Read the model definition and answer for the solid it produces. Units are mm, in the model's axes. A direction names the side the tool comes from. Coordinates: 2 decimals unless noted, no trailing zeros. Write each loop counter-clockwise with the first axis right and the second up, starting at its lowest first coordinate (ties: lowest second). Pieces come first, ordered by that corner, then holes. Notation, with made-up numbers: (-15.75, -29) -> (9.25, -29) arc R34 ccw to (9.25, 8) -> close; hole circle Ø10 at (-14, 41). An arc over 180 degrees is marked (long way). Use CSV: the item, a comma, the result in double quotes.
from build123d import *

# Parameters (mm, degrees)
BOSS_EXTRUDE2_DEPTH   = 22
BOSS_EXTRUDE3_DEPTH   = 64
SKETCH3_R             = 3
CUT_EXTRUDE1_DEPTH    = 65
SKETCH4_R             = 6
CUT_EXTRUDE2_DEPTH    = 52
M4_TAPPED_HOLE1_D     = 3.3
M4_TAPPED_HOLE1_DEPTH = 14
M4_TAPPED_HOLE1_TIP   = 0.991420021
SKETCH8_R             = 2.5
SKETCH8_R_2           = 1.5
CUT_EXTRUDE3_DEPTH    = 5
SKETCH9_R             = 1
CUT_EXTRUDE4_DEPTH    = 15
CHAMFER1_SIZE         = 1


with BuildPart() as part:
    # Sketch1 → Boss-Extrude2 (new body)
    with BuildSketch(Plane(origin=(0, 0, 0), x_dir=(1, 0, 0), z_dir=(0, 1, 0))):
        with BuildLine():
            Line((-3.31662479, -5), (3.31662479, -5))
            ThreePointArc((3.31662479, -5), (0, 6), (-3.31662479, -5))
        make_face()
    extrude(amount=BOSS_EXTRUDE2_DEPTH)

    # Sketch2 → Boss-Extrude3 (add)
    with BuildSketch(Plane(origin=(0, 22, 0), x_dir=(1, 0, 0), z_dir=(0, 1, 0))):
        with BuildLine():
            Line((-13, 7.483314774), (-13, -7.483314774))
            ThreePointArc((-13, -7.483314774), (15, 0), (-13, 7.483314774))
        make_face()
    extrude(amount=BOSS_EXTRUDE3_DEPTH)

    # Sketch3 → Cut-Extrude1 (cut)
    with BuildSketch(Plane(origin=(0, 86, 0), x_dir=(1, 0, 0), z_dir=(0, 1, 0))):
        with Locations(Location((-8, 0, 0), (0, 0, 270))):
            Circle(SKETCH3_R)
    extrude(amount=-CUT_EXTRUDE1_DEPTH, mode=Mode.SUBTRACT)

    # Sketch4 → Cut-Extrude2 (cut)
    with BuildSketch(Plane(origin=(0, 86, 0), x_dir=(1, 0, 0), z_dir=(0, 1, 0))):
        with Locations(Location((5, 0, 0), (0, 0, 270))):
            Circle(SKETCH4_R)
    extrude(amount=-CUT_EXTRUDE2_DEPTH, mode=Mode.SUBTRACT)

    # M4 Tapped Hole1
    with Locations(Plane(origin=(0, 86, 0), x_dir=(1, 0, 0), z_dir=(0, 1, 0))):
        with Locations((0, -9), (0, 9)):
            Hole(M4_TAPPED_HOLE1_D / 2, depth=M4_TAPPED_HOLE1_DEPTH)
            with Locations((0, 0, -(M4_TAPPED_HOLE1_DEPTH + M4_TAPPED_HOLE1_TIP / 2))):  # 118° drill point
                Cone(0, M4_TAPPED_HOLE1_D / 2, M4_TAPPED_HOLE1_TIP, mode=Mode.SUBTRACT)

    # Sketch8 → Cut-Extrude3 (cut)
    with BuildSketch(Plane.ZY.offset(13)):
        with Locations((0, 54)):
            Circle(SKETCH8_R)
        with Locations((0, 25)):
            Circle(SKETCH8_R_2)
    extrude(amount=-CUT_EXTRUDE3_DEPTH, mode=Mode.SUBTRACT)

    # Sketch9 → Cut-Extrude4 (cut)
    with BuildSketch(Plane.ZY.offset(13)):
        with Locations((0, 76)):
            Circle(SKETCH9_R)
        with Locations((0, 34)):
            Circle(SKETCH9_R)
    extrude(amount=-CUT_EXTRUDE4_DEPTH, mode=Mode.SUBTRACT)

    # Chamfer1
    chamfer1_edges = [part.edges().sort_by_distance(p)[0] for p in [
        (0, 0, -6),
    ]]
    chamfer(chamfer1_edges, length=CHAMFER1_SIZE - 0.0001)  # a hair under: the kernel refuses the full size


solid = part.part
1. A cutting plane is placed at C-C (z = 12). Give the vertices of the cut face in (x, y), and give its area (3 significant figures).
Solutions:
outline,"(-9, 22) -> (9, 22) -> (9, 86) -> (-9, 86) -> close"
area,"1,150 mm^2"
2. A tool of negligible diameter and unlimited length cuts with its end or side. For faces 4 (the flat face through (5, 34, 0)), 5 (the flat face through (0, 11, 5)), 6 (the cylindrical face through (0, 11, -6)), 7 (the cylindrical face through (-11.82, 25.45, 1.43)), from which of +Z, -Z, +X, -X, +Y, -Y can it reach the whole face along a straight path? Write none if from no direction.
Solutions:
face 4,"+Y"
face 5,"+Z, +X, -X, -Y"
face 6,"-Y"
face 7,"-X"
3. For a pull along Y with two mould halves and no side action, classify faces 1 (the flat face through (-13, 54, -3)), 2 (the flat face through (7, 22, 0)), 3 (the cylindrical face through (-12, 77, 0)) as pulls with the +Y half, pulls with the -Y half, needs draft (parallel to the pull), parting line crosses it, or undercut.
Solutions:
face 1,"needs draft"
face 2,"pulls with the -Y half"
face 3,"undercut"
4. Find the intervals of material crossed by line 1 along Y through (x, z) = (-12.1, 0); line 2 along Y through (x, z) = (-11.25, 8); line 3 along Y through (x, z) = (-0.75, 1.5), in increasing order.
Solutions:
line 1,"y = 22 to 23.5, 26.5 to 33, 35 to 51.5, 56.5 to 75, 77 to 86"
line 2,"y = 22 to 86"
line 3,"y = 0 to 34"
5. A cutting plane is placed at A-A (z = 0). Give the number of separate pieces and of enclosed holes in the cut face, and give its area (3 significant figures).
Solutions:
separate pieces,"8"
enclosed holes,"0"
area,"1,000 mm^2"
6. A cutting plane is placed at B-B (y = 65.5). Give the vertices of the cut face in (x, z).
Solutions:
outline,"(-13, -7.48) arc R15 ccw (long way) to (-13, 7.48) -> close; hole circle Ø6 at (-8, 0); hole circle Ø12 at (5, 0)"
7. Each of these flat-tipped pins is pushed along its axis until it touches: pin 1 Ø1.5 at (y, z) = (51, 10) entering from -X; pin 2 Ø1 at (x, z) = (9, 9.5) entering from -Y; pin 3 Ø1.8 at (y, z) = (34, 0) entering from -X. Where does it stop, or does it pass through?
Solutions:
pin 1,"stops at x = -11.81"
pin 2,"stops at y = 22"
pin 3,"stops at x = 2"
